Design review of the part built by this model. Coordinates are the model's own, in mm. A direction names the side the tool comes from. Give positions to 0.01 mm unless a question says otherwise; leave off trailing zeros. Order: outer loops, then holes, each group sorted by start corner. A loop starts at its lowest first (then second) coordinate and runs counter-clockwise, first axis right, second up. Notation, with made-up numbers: (-22.75, -35) -> (-18.75, -35) arc R19 cw to (-18.75, -26) -> close; hole circle Ø4 at (-16.5, 14). An arc over 180 degrees is marked (long way). Use a Markdown table: item, result. Add a question column.
```python
from build123d import *

# Parameters (mm, degrees)
SKETCH1_R           = 1.549999999
BOSS_EXTRUDE1_DEPTH = 6.35


with BuildPart() as part:
    # Sketch1 → Boss-Extrude1 (new body)
    with BuildSketch(Plane.XY):
        with BuildLine():
            Line((231.100613802, 220.383854223), (231.100613802, 226.717998483))
            ThreePointArc((231.100613802, 226.717998483), (231.304344536, 227.804680676), (231.887865928, 228.743769162))
            Line((231.887865928, 228.743769162), (232.144361676, 229.023939287))
            ThreePointArc((232.144361676, 229.023939287), (232.727883068, 229.963027773), (232.931613801, 231.049709965))
            Line((232.931613801, 231.049709965), (232.931613801, 234.717998484))
            ThreePointArc((232.931613801, 234.717998484), (232.727883068, 235.804680676), (232.144361676, 236.743769162))
            Line((232.144361676, 236.743769162), (231.887865928, 237.023939287))
            ThreePointArc((231.887865928, 237.023939287), (231.304344536, 237.963027773), (231.100613802, 239.049709966))
            Line((231.100613802, 239.049709966), (231.100613802, 245.383854224))
            ThreePointArc((231.100613802, 245.383854224), (232.565079896, 248.91938813), (236.100613802, 250.383854224))
            Line((236.100613802, 250.383854224), (340.100613803, 250.383854224))
            ThreePointArc((340.100613803, 250.383854224), (343.636147709, 248.919388129), (345.100613803, 245.383854222))
            Line((345.100613803, 245.383854222), (345.100613803, 220.383854223))
            ThreePointArc((345.100613803, 220.383854223), (343.636147709, 216.848320317), (340.100613803, 215.383854223))
            Line((340.100613803, 215.383854223), (236.100613802, 215.383854223))
            ThreePointArc((236.100613802, 215.383854223), (232.565079896, 216.848320317), (231.100613802, 220.383854223))
        make_face()
        with Locations((271.837613804, 228.153854225)):
            Circle(SKETCH1_R, mode=Mode.SUBTRACT)
        with Locations((283.150613802, 239.467854223)):
            Circle(SKETCH1_R, mode=Mode.SUBTRACT)
        with BuildLine():
            Line((339.550613803, 220.333854223), (336.650613802, 220.333854223))
            ThreePointArc((336.650613802, 220.333854223), (334.100613802, 222.883854224), (336.650613802, 225.433854224))
            Line((336.650613802, 225.433854224), (339.550613803, 225.433854224))
            ThreePointArc((339.550613803, 225.433854224), (342.100613803, 222.883854224), (339.550613803, 220.333854223))
        make_face(mode=Mode.SUBTRACT)
        with BuildLine():
            Line((236.650613802, 220.333854223), (239.550613804, 220.333854223))
            ThreePointArc((239.550613804, 220.333854223), (242.100613804, 222.883854224), (239.550613804, 225.433854224))
            Line((239.550613804, 225.433854224), (236.650613802, 225.433854224))
            ThreePointArc((236.650613802, 225.433854224), (234.100613802, 222.883854224), (236.650613802, 220.333854223))
        make_face(mode=Mode.SUBTRACT)
        with BuildLine():
            Line((239.550613804, 240.333854223), (236.650613802, 240.333854223))
            ThreePointArc((236.650613802, 240.333854223), (234.100613802, 242.883854224), (236.650613802, 245.433854224))
            Line((236.650613802, 245.433854224), (239.550613804, 245.433854224))
            ThreePointArc((239.550613804, 245.433854224), (242.100613804, 242.883854224), (239.550613804, 240.333854223))
        make_face(mode=Mode.SUBTRACT)
        with BuildLine():
            Line((336.650613802, 240.333854223), (339.550613803, 240.333854223))
            ThreePointArc((339.550613803, 240.333854223), (342.100613803, 242.883854224), (339.550613803, 245.433854224))
            Line((339.550613803, 245.433854224), (336.650613802, 245.433854224))
            ThreePointArc((336.650613802, 245.433854224), (334.100613802, 242.883854224), (336.650613802, 240.333854223))
        make_face(mode=Mode.SUBTRACT)
    extrude(amount=BOSS_EXTRUDE1_DEPTH)


solid = part.part
```
1) Machinability: for faces 4 (the flat face through (231.101, 224, 3)), 5 (the cylindrical face through (242.1, 242.9, 3.1)), 6 (the cylindrical face through (232.722, 229.949, 3.131)), which of the approach directions +Z, -Z, +X, -X, +Y, -Y give a long, thin tool a straight path to every point of the face, cutting with its end or side? Answer none if there is none.
2) Add section B-B (y = 221.5). Give the boundary of the cut face in (x, z).
3) For L1, parallel to Y at x = 337.5, z = 1.5; L2, parallel to X at y = 221.5, z = 2.5; L3, parallel to X at y = 224.5, z = 3, list the stretches that pass through material, from the lowest coordinate up. Write a range as [from, to].
4) Insertion check: pin 1 (3 mm diameter, centred on y = 233.5, z = 2, fed in from -X); pin 2 (3 mm diameter, centred on y = 229.5, z = 1, fed in from -X). Each pin has a flat end and moves straight along its axis. Give the tip position at first contact, or say it passes through.
5) Add section A-A (x = 338). Give the boundary of the cut face in (y, z).
6) The part is to be moulded in two halves that separate along Y. For faces 1 (the cylindrical face through (231.31, 237.95, 3.13)), 2 (the cylindrical face through (343.597, 248.958, 3.131)), 3 (the flat face through (289, 233, 6.35)), say which applies: +Y half, -Y half, draft (parallel to the pull), parting line (faces both ways), or undercut.
7) Add section C-C (z = 2.75). Give the number of separate pieces and of enclosed holes in the cut face, then the cut area to 3 significant figures.
Worked answers:
| question | item | result |
|---|---|---|
| 1 | face 4 | +Z, -Z, -X, +Y, -Y |
| 1 | face 5 | +Z, -Z |
| 1 | face 6 | +Z, -Z, -X |
| 2 | outline | (231.1, 0) -> (234.51, 0) -> (234.51, 6.35) -> (231.1, 6.35) -> close; (241.69, 0) -> (334.51, 0) -> (334.51, 6.35) -> (241.69, 6.35) -> close; (341.69, 0) -> (345.1, 0) -> (345.1, 6.35) -> (341.69, 6.35) -> close |
| 3 | L1 | [215.38, 220.33], [225.43, 240.33], [245.43, 250.38] |
| 3 | L2 | [231.1, 234.51], [241.69, 334.51], [341.69, 345.1] |
| 3 | L3 | [231.1, 234.68], [241.52, 334.68], [341.52, 345.1] |
| 4 | pin 1 | x = 232.92 |
| 4 | pin 2 | x = 231.39 |
| 5 | outline | (215.38, 0) -> (220.33, 0) -> (220.33, 6.35) -> (215.38, 6.35) -> close; (225.43, 0) -> (240.33, 0) -> (240.33, 6.35) -> (225.43, 6.35) -> close; (245.43, 0) -> (250.38, 0) -> (250.38, 6.35) -> (245.43, 6.35) -> close |
| 6 | face 1 | undercut |
| 6 | face 2 | +Y half |
| 6 | face 3 | draft |
| 7 | separate pieces | 1 |
| 7 | enclosed holes | 6 |
| 7 | area | 3,800 mm^2 |
